For this review, take the finished solid that the model builds, in its own axes (mm). A direction names the side the tool comes from. Give positions to 0.01 mm unless a question says otherwise; leave off trailing zeros. Write each loop counter-clockwise with the first axis right and the second up, starting at its lowest first coordinate (ties: lowest second). Pieces come first, ordered by that corner, then holes. Notation, with made-up numbers: M 13,9.5 L 42,9.5 A22 cw 42,15.5 Z; hole C 22,23.25 d6. An arc over 180 degrees is marked long. Use one line per item in the form item = value. Start each with the question number.
Q1. Tool access review of faces 1 (the flat face through (-5.474, 39.132, -3.219)), 2 (the cylindrical face through (-1.8, 66.5, -0.6)): name each direction out of +Z, -Z, +X, -X, +Y, -Y from which nothing blocks a thin tool from reaching the whole face with its end or side.
Q2. Consider section B-B on y = 70.5. Write out the cut boundary in (x, z), and give its area (3 significant figures).
Q3. Mouldability with a two-part tool opening along X and no side actions: class faces 3 (the flat face through (5.525, 39.132, -3.131)), 4 (the conical face through (0.177, 53.032, -0.278)), 5 (the cylindrical face through (-1.02, 27, -0.09)), 6 (the flat face through (0, 39, -6.35)) as released by +X, released by -X, zero draft, split by the parting line, or undercut.
Q4. Consider section C-C on z = 3.5. Write out the cut boundary in (x, y) (3 decimals), and give its area (3 significant figures).
Q5. Clearance check with flat-ended pins moving along their axes: pin 1 Ø2 at (x, z) = (-2.5, 3.5) entering from -Y; pin 2 Ø6 at (y, z) = (20.5, 4.5) entering from +X; pin 3 Ø2.5 at (x, y) = (0, 25.4) entering from +Z; pin 4 Ø2 at (y, z) = (33, 0.5) entering from +X. State where each tip first meets the part, or that it passes through.
Q6. Consider section A-A on y = 25.4. Write out the cut boundary in (x, z), and give its area (3 significant figures).
Q7. For probe 1 along Z at (x, y) = (0, 63.75); probe 2 along Y at (x, z) = (0, -2.5) (3 decimals); probe 3 along Z at (x, y) = (1, 73), list the stretches that pass through material, from the lowest coordinate up. Write a range as [from, to].
Q8. Consider section D-D on y = 14. Write out the cut boundary in (x, z).
```python
from build123d import *

# Parameters (mm, degrees)
BOSS_EXTRUDE1_DEPTH            = 79.375
TAP_DRILL_FOR_10_24_TAP1_D     = 3.7973
TAP_DRILL_FOR_10_24_TAP1_DEPTH = 25.4
TAP_DRILL_FOR_10_24_TAP1_TIP   = 1.140824014
TAP_DRILL_FOR_10_24_TAP2_D     = 3.7973
TAP_DRILL_FOR_10_24_TAP2_DEPTH = 25.4
TAP_DRILL_FOR_10_24_TAP2_TIP   = 1.140824014


with BuildPart() as part:
    # Sketch1 → Boss-Extrude1 (new body)
    with BuildSketch(Plane(origin=(0, 0, 0), x_dir=(1, 0, 0), z_dir=(0, 1, 0))):
        Polygon((7.332348419, 0), (3.666174209, 6.35), (-3.666174209, 6.35), (-7.332348419, 0), (-3.666174209, -6.35), (3.666174209, -6.35), align=None)
    extrude(amount=BOSS_EXTRUDE1_DEPTH)

    # Tap Drill for #10-24 Tap1
    with Locations(Plane(origin=(0, 79.375, 0), x_dir=(1, 0, 0), z_dir=(0, 1, 0))):
        with Locations((0, 0)):
            Hole(TAP_DRILL_FOR_10_24_TAP1_D / 2, depth=TAP_DRILL_FOR_10_24_TAP1_DEPTH)
            with Locations((0, 0, -(TAP_DRILL_FOR_10_24_TAP1_DEPTH + TAP_DRILL_FOR_10_24_TAP1_TIP / 2))):  # 118° drill point
                Cone(0, TAP_DRILL_FOR_10_24_TAP1_D / 2, TAP_DRILL_FOR_10_24_TAP1_TIP, mode=Mode.SUBTRACT)

    # Tap Drill for #10-24 Tap2
    with Locations(Plane.XY.offset(6.35)):
        with Locations((0, 25.4)):
            Hole(TAP_DRILL_FOR_10_24_TAP2_D / 2, depth=TAP_DRILL_FOR_10_24_TAP2_DEPTH)
            with Locations((0, 0, -(TAP_DRILL_FOR_10_24_TAP2_DEPTH + TAP_DRILL_FOR_10_24_TAP2_TIP / 2))):  # 118° drill point
                Cone(0, TAP_DRILL_FOR_10_24_TAP2_D / 2, TAP_DRILL_FOR_10_24_TAP2_TIP, mode=Mode.SUBTRACT)


solid = part.part
```
Working result:
q1.face_1 = -Z, -X, +Y, -Y
q1.face_2 = +Y
q2.outline = M -7.33,0 L -3.67,-6.35 L 3.67,-6.35 L 7.33,0 L 3.67,6.35 L -3.67,6.35 Z; hole C 0,0 d3.8
q2.area = 128 mm²
q3.face_3 = released by +X
q3.face_4 = undercut
q3.face_5 = undercut
q3.face_6 = zero draft
q4.outline = M -5.312,0 L 5.312,0 L 5.312,79.375 L -5.312,79.375 Z; hole C 0,25.4 d3.797
q4.area = 832 mm²
q5.pin_1 = 0
q5.pin_2 = 6.47
q5.pin_3 = through
q5.pin_4 = 7.33
q6.outline = M -7.33,0 L -3.67,-6.35 L -1.9,-6.35 L -1.9,6.35 L -3.67,6.35 Z; M 1.9,-6.35 L 3.67,-6.35 L 7.33,0 L 3.67,6.35 L 1.9,6.35 Z
q6.area = 91.5 mm²
q7.probe_1 = [-6.35, -1.9], [1.9, 6.35]
q7.probe_2 = [0, 23.501], [27.299, 79.375]
q7.probe_3 = [-6.35, -1.61], [1.61, 6.35]
q8.outline = M -7.33,0 L -3.67,-6.35 L 3.67,-6.35 L 7.33,0 L 3.67,6.35 L -3.67,6.35 Z
